```python
from build123d import *

# Parameters (mm, degrees)
SKETCH1_W               = 150
SKETCH1_H               = 73
BOSS_EXTRUDE1_DEPTH     = 3
SKETCH2_W               = 3
SKETCH2_H               = 10
CUT_EXTRUDE1_DEPTH      = 84.464064123
LPATTERN1_COUNT         = 4
LPATTERN1_PITCH         = 20
MIRROR3_COPY_1_SKETCH_W = 3
MIRROR3_COPY_1_SKETCH_H = 10
MIRROR3_COPY_1_DEPTH    = 84.464064123
MIRROR3_COPY_2_SKETCH_W = 3
MIRROR3_COPY_2_SKETCH_H = 10
MIRROR3_COPY_2_DEPTH    = 84.464064123
MIRROR3_COPY_3_SKETCH_W = 3
MIRROR3_COPY_3_SKETCH_H = 10
MIRROR3_COPY_3_DEPTH    = 84.464064123
SKETCH4_W               = 10
SKETCH4_H               = 3
CUT_EXTRUDE3_DEPTH      = 84.464064123
LPATTERN2_COUNT         = 8
LPATTERN2_PITCH         = 20
SKETCH5_W               = 10
SKETCH5_H               = 3
CUT_EXTRUDE4_DEPTH      = 84.464064123
LPATTERN4_COUNT         = 7
LPATTERN4_PITCH         = 20
SKETCH6_W               = 120
SKETCH6_H               = 20
CUT_EXTRUDE5_DEPTH      = 84.464064123
FILLET1_R               = 10


with BuildPart() as part:
    # Sketch1 → Boss-Extrude1 (new body)
    with BuildSketch(Plane.XY):
        Rectangle(SKETCH1_W, SKETCH1_H)
    extrude(amount=BOSS_EXTRUDE1_DEPTH)

    # Sketch2 → Cut-Extrude1 (cut, through all)
    with BuildSketch(Plane.XY.offset(3)):
        with Locations((-73.5, 21.5)):
            Rectangle(SKETCH2_W, SKETCH2_H)
    cut_extrude1 = extrude(amount=-CUT_EXTRUDE1_DEPTH, mode=Mode.SUBTRACT)

    # LPattern1: Cut-Extrude1 ×4
    with Locations(*[(0, -i * LPATTERN1_PITCH, 0) for i in range(1, LPATTERN1_COUNT)]):
        add(cut_extrude1, mode=Mode.SUBTRACT)

    # Mirror3: Cut-Extrude1 across plane
    add(cut_extrude1.mirror(Plane(origin=(0, 0, 0), x_dir=(0, 0, 1), z_dir=(1, 0, 0))), mode=Mode.SUBTRACT)

    # Mirror3 copy 1 sketch → Mirror3 copy 1 (cut, through all)
    with BuildSketch(Plane(origin=(0, -20, 3), x_dir=(-1, 0, 0), z_dir=(0, 0, 1))):
        with Locations((-73.5, -21.5)):
            Rectangle(MIRROR3_COPY_1_SKETCH_W, MIRROR3_COPY_1_SKETCH_H)
    extrude(amount=-MIRROR3_COPY_1_DEPTH, mode=Mode.SUBTRACT)

    # Mirror3 copy 2 sketch → Mirror3 copy 2 (cut, through all)
    with BuildSketch(Plane(origin=(0, -40, 3), x_dir=(-1, 0, 0), z_dir=(0, 0, 1))):
        with Locations((-73.5, -21.5)):
            Rectangle(MIRROR3_COPY_2_SKETCH_W, MIRROR3_COPY_2_SKETCH_H)
    extrude(amount=-MIRROR3_COPY_2_DEPTH, mode=Mode.SUBTRACT)

    # Mirror3 copy 3 sketch → Mirror3 copy 3 (cut, through all)
    with BuildSketch(Plane(origin=(0, -60, 3), x_dir=(-1, 0, 0), z_dir=(0, 0, 1))):
        with Locations((-73.5, -21.5)):
            Rectangle(MIRROR3_COPY_3_SKETCH_W, MIRROR3_COPY_3_SKETCH_H)
    extrude(amount=-MIRROR3_COPY_3_DEPTH, mode=Mode.SUBTRACT)

    # Sketch4 → Cut-Extrude3 (cut, through all)
    with BuildSketch(Plane.XY.offset(3)):
        with Locations((60, -35)):
            Rectangle(SKETCH4_W, SKETCH4_H)
    cut_extrude3 = extrude(amount=-CUT_EXTRUDE3_DEPTH, mode=Mode.SUBTRACT)

    # LPattern2: Cut-Extrude3 ×8
    with Locations(*[(-i * LPATTERN2_PITCH, 0, 0) for i in range(1, LPATTERN2_COUNT)]):
        add(cut_extrude3, mode=Mode.SUBTRACT)

    # Sketch5 → Cut-Extrude4 (cut, through all)
    with BuildSketch(Plane.XY.offset(3)):
        with Locations((-60, 10)):
            Rectangle(SKETCH5_W, SKETCH5_H)
    cut_extrude4 = extrude(amount=-CUT_EXTRUDE4_DEPTH, mode=Mode.SUBTRACT)

    # LPattern4: Cut-Extrude4 ×7
    with Locations(*[(i * LPATTERN4_PITCH, 0, 0) for i in range(1, LPATTERN4_COUNT)]):
        add(cut_extrude4, mode=Mode.SUBTRACT)

    # Sketch6 → Cut-Extrude5 (cut, through all)
    with BuildSketch(Plane.XY.offset(3)):
        with Locations((0, -11.5)):
            Rectangle(SKETCH6_W, SKETCH6_H)
    extrude(amount=-CUT_EXTRUDE5_DEPTH, mode=Mode.SUBTRACT)

    # Fillet1
    fillet1_edges = [part.edges().sort_by_distance(p)[0] for p in [
        (60, -1.5, 1.5),
        (60, -21.5, 1.5),
        (-60, -1.5, 1.5),
        (-60, -21.5, 1.5),
    ]]
    fillet(fillet1_edges, radius=FILLET1_R - 0.0001)  # a hair under: the kernel refuses the full size


solid = part.part
```
The model under review builds one solid part; all positions refer to its coordinate system, in mm. A direction names the side the tool comes from. Round coordinates to 2 decimals unless told otherwise and drop trailing zeros. Order: outer loops, then holes, each group sorted by start corner. A loop starts at its lowest first (then second) coordinate and runs counter-clockwise, first axis right, second up. Notation, with made-up numbers: M -0.75,-19 L 53.25,-19 A16 ccw 53.25,-9 Z; hole C 52.25,87 d6. An arc over 180 degrees is marked long. Use a Markdown table: item, result.
1) Tool access review of faces 3 (the face through (-55, -35, 2)), 4 (the face through (-74, 16.5, 2)), 5 (the face through (40, 11.5, 2)), 6 (the face through (74, 16.5, 2)), 7 (the face through (-30, -36.5, 1)): name each direction out of +Z, -Z, +X, -X, +Y, -Y from which nothing blocks a thin tool from reaching the whole face with its end or side.
Report:
| item | result |
|---|---|
| face 3 | +Z, -Z, -Y |
| face 4 | +Z, -Z, -X |
| face 5 | +Z, -Z |
| face 6 | +Z, -Z, +X |
| face 7 | +Z, -Z, +X, -X, -Y |
2) Insertion check: pin 1 (1.5 mm diameter, centred on x = -73.5, z = 1.5, fed in from -Y); pin 2 (1.5 mm diameter, centred on y = 2.5, z = 1.5, fed in from +X); pin 3 (0.9 mm diameter, centred on y = -34.5, z = 1, fed in from -X). Each pin has a flat end and moves straight along its axis. Give the tip position at first contact, or say it passes through.
Report:
| item | result |
|---|---|
| pin 1 | y = -33.5 |
| pin 2 | x = 72 |
| pin 3 | x = -72 |
3) Consider section C-C (z = 2.1). Give the number of separate pieces and of enclosed holes in the cut face, then the cut area to 3 significant figures.
Report:
| item | result |
|---|---|
| separate pieces | 1 |
| enclosed holes | 8 |
| area | 8,020 mm^2 |
4) Draft analysis for pull direction X (two halves, no side actions). For faces 1 (the face through (-74, -3.5, 2)), 2 (the face through (45, 10, 2)), state which applies: released by +X, released by -X, zero draft, split by the parting line, or undercut.
Report:
| item | result |
|---|---|
| face 1 | zero draft |
| face 2 | undercut |
5) Consider section A-A (x = -6.5). Write out the cut boundary in (y, z), then the cut area to 3 significant figures.
Report:
| item | result |
|---|---|
| outline | M -36.5,0 L -21.5,0 L -21.5,3 L -36.5,3 Z; M -1.5,0 L 36.5,0 L 36.5,3 L -1.5,3 Z |
| area | 159 mm^2 |
6) Wall thickness on line 1 along Y through (x, z) = (-24.5, 1.1); line 2 along Y through (x, z) = (-34, 2.1); line 3 along Y through (x, z) = (-64, 1.2): over which ranges is each line inside the solid? List them lowest first. Write a range as [from, to].
Report:
| item | result |
|---|---|
| line 1 | [-33.5, -21.5], [-1.5, 8.5], [11.5, 36.5] |
| line 2 | [-36.5, -21.5], [-1.5, 36.5] |
| line 3 | [-33.5, 8.5], [11.5, 36.5] |
7) Consider section B-B (y = 2). Write out the cut boundary in (x, z).
Report:
| item | result |
|---|---|
| outline | M -72,0 L 72,0 L 72,3 L -72,3 Z |
